Model file for the job. Use its own axes, mm. A direction names the side the tool comes from. Give positions to 0.01 mm unless a question says otherwise; leave off trailing zeros. Order: outer loops, then holes, each group sorted by start corner. A loop starts at its lowest first (then second) coordinate and runs counter-clockwise, first axis right, second up. Notation, with made-up numbers: M 62.25,-34.5 L 109.25,-34.5 A28 cw 109.25,-0.5 Z; hole C 35.5,-3 d7. An arc over 180 degrees is marked long. Return JSON: item names as keys, results as strings. Group by question number.
1. Slice it at B-B on z = 19. List the corners of the cut face in (x, y), then the cut area to 3 significant figures.
2. Wall check: probe 1 along Y at (x, z) = (-41.5, 5); probe 2 along Y at (x, z) = (-43, 8.5); probe 3 along Z at (x, y) = (-40, -11). Give the ranges that are in metal, low to high. Write a range as [from, to].
3. Pin check, flat tips, straight feed: pin 1 (4 mm diameter, centred on x = -37.5, z = 16.5, fed in from -Y); pin 2 (5 mm diameter, centred on y = -5.5, z = 33, fed in from -X); pin 3 (4 mm diameter, centred on x = -37, z = 17.5, fed in from +Y). Stop position of each tip, or through.
4. 3-axis set-ups, long thin cutter, end or side, ignore diameter. For faces 1 (the face through (-27.254, 4.552, 31.363)), 2 (the face through (-46, 5, 12.993)): which of +Z, -Z, +X, -X, +Y, -Y reach the whole face in a straight line?
5. Slice it at A-A on z = 5. List the corners of the cut face in (x, y).
6. Two-plate mould, pull along Z, no slides. Class faces 3 (the face through (-42, 0, -11.423)), 4 (the face through (-42, 0, 43.835)), 5 (the face through (-48.127, 0.283, 7.332)): released by +Z, released by -Z, zero draft, split by the parting line, or undercut.
from build123d import *

# Parameters (mm, degrees)
F2_R = 1.5912908075
F3_R = 21.8711796934


with BuildPart() as f1:
    # F0 (on Front) → F1 (revolve)
    with BuildSketch(Plane.XZ):
        Polygon((-30.3995665163, 43.8347905874), (-41.7082160711, 43.8347905874), (-41.7082160711, -11.4233754575), (-31.1706103384, -11.4233754575), (-35.2828465402, -4.483976867), (-35.2828465402, 12.9930237308), (-20.8900216967, 12.9930237308), align=None)
    revolve(axis=Axis((-41.7082160711, 0, 16.2057075649), (0, 0, 1)))

    # F2
    f2_edges = [f1.edges().sort_by_distance(p)[0] for p in [
        (-53.016866, 0, 43.834791),
    ]]
    fillet(f2_edges, radius=F2_R)

    # F3
    f3_edges = [f1.edges().sort_by_distance(p)[0] for p in [
        (-48.133586, 0, -4.483977),
    ]]
    fillet(f3_edges, radius=F3_R)


solid = f1.part
Result:
{
 "1": {"outline": "C -41.71,0 d37.93", "area": "1,130 mm2"},
 "2": {"probe 1": "y = [-6.42, 6.42]", "probe 2": "y = [-6.29, 6.29]", "probe 3": "z = [12.99, 43.48]"},
 "3": {"pin 1": "stops at y = -20.02", "pin 2": "stops at x = -56.44", "pin 3": "stops at y = 19.62"},
 "4": {"face 1": "+Z", "face 2": "none"},
 "5": {"outline": "C -41.71,0 d12.85"},
 "6": {"face 3": "released by -Z", "face 4": "released by +Z", "face 5": "undercut"}
}
